Work out the finished part from the listing and answer in its coordinate system (mm). A direction names the side the tool comes from. Give positions to 0.01 mm unless a question says otherwise; leave off trailing zeros. Loops run counter-clockwise (first coordinate to the right, second up) from the corner with the lowest first, then second, coordinate; pieces in that order, holes last. Notation, with made-up numbers: M 48.25,-39.75 L 88.25,-39.75 A22 cw 88.25,-13.75 Z; hole C -19.5,-10.75 d1. An arc over 180 degrees is marked long. Answer as a JSON object with one key per item and string values. Group by question number.
```python
from build123d import *

# Parameters (mm, degrees)
SKETCH2_R           = 1.35
BOSS_EXTRUDE1_DEPTH = 8.5
CUT_EXTRUDE1_DEPTH  = 6.4
CUT_EXTRUDE2_DEPTH  = 3.2
SKETCH6_R           = 3
BOSS_EXTRUDE2_DEPTH = 1


with BuildPart() as part:
    # Sketch2 → Boss-Extrude1 (new body, symmetric)
    with BuildSketch(Plane.XY):
        Circle(SKETCH2_R)
    extrude(amount=BOSS_EXTRUDE1_DEPTH, both=True)

    # Sketch4 → Cut-Extrude1 (cut)
    with BuildSketch(Plane(origin=(0, 0, -8.5), x_dir=(-1, 0, 0), z_dir=(0, 0, -1))):
        with BuildLine():
            Line((1, 0.906917857), (1, -0.906917857))
            ThreePointArc((1, -0.906917857), (1.35, 0), (1, 0.906917857))
        make_face()
    extrude(amount=-CUT_EXTRUDE1_DEPTH, mode=Mode.SUBTRACT)

    # Sketch5 → Cut-Extrude2 (cut)
    with BuildSketch(Plane.XY.offset(8.5)):
        with BuildLine():
            Line((-1, 0.906917857), (-1, -0.906917857))
            ThreePointArc((-1, -0.906917857), (-1.35, 0), (-1, 0.906917857))
        make_face()
    extrude(amount=-CUT_EXTRUDE2_DEPTH, mode=Mode.SUBTRACT)

    # Sketch6 → Boss-Extrude2 (add)
    with BuildSketch(Plane(origin=(0, 0, -8.5), x_dir=(-1, 0, 0), z_dir=(0, 0, -1))):
        Circle(SKETCH6_R)
    extrude(amount=BOSS_EXTRUDE2_DEPTH)


solid = part.part
```
Item 1: A cutting plane is placed at C-C (z = -3.5). Determine the outline of the cut face in (x, y), and give its area (3 significant figures).
Item 2: A cutting plane is placed at A-A (x = 0). Determine the outline of the cut face in (y, z).
Item 3: Given pin 1 Ø2 at (y, z) = (0, -6) entering from -X; pin 2 Ø3 at (y, z) = (-0.5, 6.5) entering from +X, each flat-ended and moving along its own axis, determine where each tip first touches the part or whether it passes through.
Item 4: A cutting plane is placed at D-D (y = -1.9). Determine the outline of the cut face in (x, z).
Item 5: Find the intervals of material crossed by probe 1 along Y at (x, z) = (1, 2.75); probe 2 along Z at (x, y) = (2.1, -1.85); probe 3 along X at (y, z) = (0.95, 4.5), in increasing order. Write a range as [from, to].
Item 6: A cutting plane is placed at B-B (y = -0.2). Determine the outline of the cut face in (x, z), and give its area (3 significant figures).
Item 7: For a pull along Z with two mould halves and no side action, classify faces 3 (the cylindrical face through (3, 0, -9)), 4 (the flat face through (-1, 0, -5)), 5 (the flat face through (0, 0, -9.5)), 6 (the flat face through (0, 0, 8.5)) as pulls with the +Z half, pulls with the -Z half, needs draft (parallel to the pull), parting line crosses it, or undercut.
Item 8: A tool of negligible diameter and unlimited length cuts with its end or side. For faces 1 (the cylindrical face through (1.288, 0.406, 0.119)), 2 (the flat face through (-1, 0, 7)), from which of +Z, -Z, +X, -X, +Y, -Y can it reach the whole face along a straight path? Write none if from no direction.
The answers:
{
 "1": {"outline": "M -1,-0.91 A1.35 ccw long -1,0.91 Z", "area": "5.29 mm^2"},
 "2": {"outline": "M -3,-9.5 L 3,-9.5 L 3,-8.5 L 1.35,-8.5 L 1.35,8.5 L -1.35,8.5 L -1.35,-8.5 L -3,-8.5 Z"},
 "3": {"pin 1": "stops at x = -1", "pin 2": "stops at x = 1.35"},
 "4": {"outline": "M -2.32,-9.5 L 2.32,-9.5 L 2.32,-8.5 L -2.32,-8.5 Z"},
 "5": {"probe 1": "y = [-0.91, 0.91]", "probe 2": "z = [-9.5, -8.5]", "probe 3": "x = [-0.96, 0.96]"},
 "6": {"outline": "M -2.99,-9.5 L 2.99,-9.5 L 2.99,-8.5 L 1.34,-8.5 L 1.34,8.5 L -1,8.5 L -1,5.3 L -1.34,5.3 L -1.34,-2.1 L -1,-2.1 L -1,-8.5 L -2.99,-8.5 Z", "area": "48.2 mm^2"},
 "7": {"face 3": "needs draft", "face 4": "undercut", "face 5": "pulls with the -Z half", "face 6": "pulls with the +Z half"},
 "8": {"face 1": "+Z", "face 2": "+Z, -X, +Y, -Y"}
}
